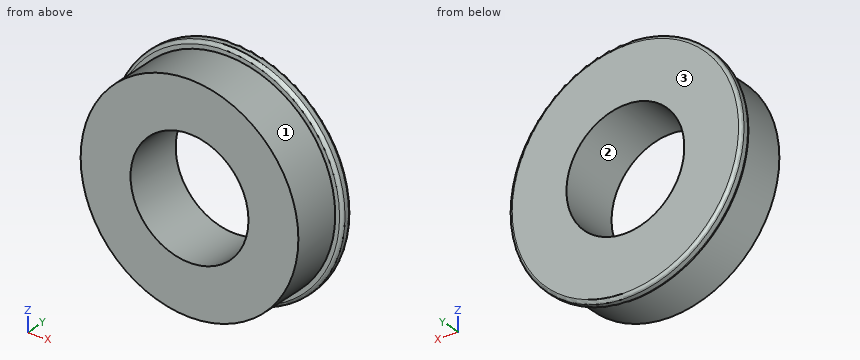
```python
from build123d import *

# Parameters (mm, degrees)
F0_R     = 17.55
F0_R_2   = 9.51
F1_DEPTH = 9.58
F2_R     = 18.75
F2_R_2   = 17.55
F3_DEPTH = 1.75
F4_R     = 0.5


with BuildPart() as f1:
    # F0 (on Front) → F1 (new body)
    with BuildSketch(Plane.XZ):
        Circle(F0_R)
        Circle(F0_R_2, mode=Mode.SUBTRACT)
    extrude(amount=F1_DEPTH)

    # F2 (on Front) → F3 (join)
    with BuildSketch(Plane.XZ):
        Circle(F2_R)
        Circle(F2_R_2, mode=Mode.SUBTRACT)
    extrude(amount=F3_DEPTH)

    # F4
    f4_edges = [f1.edges().sort_by_distance(p)[0] for p in [
        (-18.75, -1.75, 0),
        (-18.75, 0, 0),
    ]]
    fillet(f4_edges, radius=F4_R)


solid = f1.part
```
Model file for the job. Use its own axes, mm. Face numbers are marked on the shaded views. Give positions to 0.01 mm unless a question says otherwise; leave off trailing zeros. Write each loop counter-clockwise with the first axis right and the second up, starting at its lowest first coordinate (ties: lowest second). Pieces come first, ordered by that corner, then holes. Notation, with made-up numbers: (34, -25.5) -> (66, -25.5) arc R33 ccw to (66, 8.5) -> close; hole circle Ø11 at (3, 2.25). An arc over 180 degrees is marked (long way). Use CSV: the item, a comma, the result in double quotes. Start each with the question number.
1) Pin check, flat tips, straight feed: P1, Ø1, axis at x = -10, y = -7, coming from the -Z side; P2, Ø1.5, axis at y = -2, z = 7, coming from the -X side; P3, Ø2, axis at y = -1.5, z = -12.5, coming from the -X side. Stop position of each tip, or through.
2) Cut at B-B on x = 0. List the corners of the cut face in (y, z), plus the area to 3 significant figures.
3) Drill centre lines: L1, parallel to Z at x = 0, y = -4.25; L2, parallel to Z at x = 4, y = -6.5; L3, parallel to X at y = -1, z = -1.5. Where is each one in solid material? Low to high.
4) Cut at C-C on y = -5.25. List the corners of the cut face in (x, z), plus the area to 3 significant figures.
5) Cut at A-A on z = 0. List the corners of the cut face in (x, y).
6) Two-plate mould, pull along Z, no slides. Class the marked faces 1, 2 and 3: released by +Z, released by -Z, zero draft, split by the parting line, or undercut.
Final values:
1,P1,"stops at z = -14.76"
1,P2,"stops at x = -17.55"
1,P3,"stops at x = -14.79"
2,outline,"(-9.58, -17.55) -> (-1.75, -17.55) -> (-1.75, -18.25) arc R0.5 ccw to (-1.25, -18.75) -> (-0.5, -18.75) arc R0.5 ccw to (0, -18.25) -> (0, -9.51) -> (-9.58, -9.51) -> close; (-9.58, 9.51) -> (0, 9.51) -> (0, 18.25) arc R0.5 ccw to (-0.5, 18.75) -> (-1.25, 18.75) arc R0.5 ccw to (-1.75, 18.25) -> (-1.75, 17.55) -> (-9.58, 17.55) -> close"
2,area,"158 mm2"
3,L1,"z = -17.55 to -9.51, 9.51 to 17.55"
3,L2,"z = -17.09 to -8.63, 8.63 to 17.09"
3,L3,"x = -18.69 to -9.39, 9.39 to 18.69"
4,outline,"circle Ø35.1 at (0, 0); hole circle Ø19.02 at (0, 0)"
4,area,"683 mm2"
5,outline,"(-18.75, -1.25) arc R0.5 ccw to (-18.25, -1.75) -> (-17.55, -1.75) -> (-17.55, -9.58) -> (-9.51, -9.58) -> (-9.51, 0) -> (-18.25, 0) arc R0.5 ccw to (-18.75, -0.5) -> close; (9.51, -9.58) -> (17.55, -9.58) -> (17.55, -1.75) -> (18.25, -1.75) arc R0.5 ccw to (18.75, -1.25) -> (18.75, -0.5) arc R0.5 ccw to (18.25, 0) -> (9.51, 0) -> close"
6,face 1,"split by the parting line"
6,face 2,"undercut"
6,face 3,"zero draft"
